Design review of the part built by this model. Coordinates are the model's own, in mm. Face numbers are marked on the shaded views. Round coordinates to 2 decimals unless told otherwise and drop trailing zeros. Write each loop counter-clockwise with the first axis right and the second up, starting at its lowest first coordinate (ties: lowest second). Pieces come first, ordered by that corner, then holes. Notation, with made-up numbers: (39.25, -34) -> (77.25, -34) arc R29 ccw to (77.25, -9) -> close; hole circle Ø10 at (27.25, 22). An arc over 180 degrees is marked (long way). One line per question, with ' | ' between items. Start each with the question number.
1) For probe 1 along X at (y, z) = (3.25, -5); probe 2 along X at (y, z) = (7.5, -6.5); probe 3 along Y at (x, z) = (20, -1.75), list the stretches that pass through material, from the lowest coordinate up.
2) Consider section A-A (z = -5). Give the boundary of the cut face in (x, y), then the cut area to 3 significant figures.
3) Consider section B-B (y = 5.6). Give the boundary of the cut face in (x, z), then the cut area to 3 significant figures.
4) Mouldability with a two-part tool opening along X and no side actions: class the marked faces 1, 2, 3 and 4 as +X half, -X half, draft (parallel to the pull), parting line (faces both ways), or undercut.
5) Consider section D-D (y = 7.75). Give the boundary of the cut face in (x, z).
6) Consider section C-C (x = 5). Give the boundary of the cut face in (y, z).
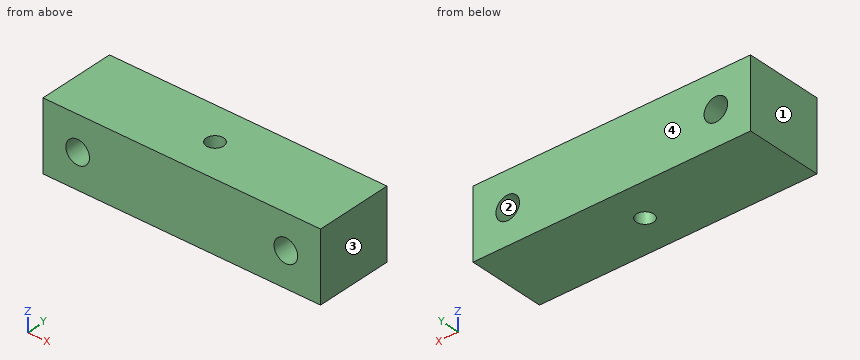
```python
from build123d import *

# Parameters (mm, degrees)
SKETCH1_W             = 40
SKETCH1_H             = 10
BOSS_EXTRUDE1_DEPTH   = 11.2
M3_CLEARANCE_HOLE1_D  = 3.4
M3X0_5_TAPPED_HOLE1_D = 2.5


with BuildPart() as part:
    # Sketch1 → Boss-Extrude1 (new body)
    with BuildSketch(Plane(origin=(0, 0, 0), x_dir=(1, 0, 0), z_dir=(0, 1, 0))):
        with Locations((20, 5)):
            Rectangle(SKETCH1_W, SKETCH1_H)
    extrude(amount=BOSS_EXTRUDE1_DEPTH)

    # M3 Clearance Hole1 (through all)
    with Locations(Plane(origin=(5, 11.2, -5), x_dir=(0, 0, 1), z_dir=(0, 1, 0))):
        with Locations((0, 0), (0, 30)):
            Hole(M3_CLEARANCE_HOLE1_D / 2)

    # M3x0.5 Tapped Hole1 (through all)
    with Locations(Plane(origin=(20, 5.6, 0), x_dir=(1, 0, 0), z_dir=(0, 0, 1))):
        with Locations((0, 0)):
            Hole(M3X0_5_TAPPED_HOLE1_D / 2)


solid = part.part
```
From the geometry:
1) probe 1: x = 0 to 3.3, 6.7 to 33.3, 36.7 to 40 | probe 2: x = 0 to 4.2, 5.8 to 34.2, 35.8 to 40 | probe 3: y = 0 to 4.35, 6.85 to 11.2
2) outline: (0, 0) -> (3.3, 0) -> (3.3, 11.2) -> (0, 11.2) -> close; (6.7, 0) -> (33.3, 0) -> (33.3, 11.2) -> (6.7, 11.2) -> close; (36.7, 0) -> (40, 0) -> (40, 11.2) -> (36.7, 11.2) -> close; hole circle Ø2.5 at (20, 5.6) | area: 367 mm2
3) outline: (0, -10) -> (18.75, -10) -> (18.75, 0) -> (0, 0) -> close; (21.25, -10) -> (40, -10) -> (40, 0) -> (21.25, 0) -> close; hole circle Ø3.4 at (5, -5); hole circle Ø3.4 at (35, -5) | area: 357 mm2
4) face 1: -X half | face 2: undercut | face 3: +X half | face 4: draft
5) outline: (0, -10) -> (40, -10) -> (40, 0) -> (0, 0) -> close; hole circle Ø3.4 at (5, -5); hole circle Ø3.4 at (35, -5)
6) outline: (0, -10) -> (11.2, -10) -> (11.2, -6.7) -> (0, -6.7) -> close; (0, -3.3) -> (11.2, -3.3) -> (11.2, 0) -> (0, 0) -> close
